The model under review builds one solid part; all positions refer to its coordinate system, in mm. Face numbers are marked on the shaded views. A direction names the side the tool comes from. Round coordinates to 2 decimals unless told otherwise and drop trailing zeros. Write each loop counter-clockwise with the first axis right and the second up, starting at its lowest first coordinate (ties: lowest second). Pieces come first, ordered by that corner, then holes. Notation, with made-up numbers: M 53.5,-9 L 105.5,-9 A16 ccw 105.5,12 Z; hole C 0,4.5 d5. An arc over 180 degrees is marked long. Write item = value, one per line. Start each with the question number.
Item 1: The part is to be moulded in two halves that separate along X. For the marked faces 4, 5 and 6, say which applies: +X half, -X half, draft (parallel to the pull), parting line (faces both ways), or undercut.
Item 2: Take a section at A-A, the plane x = 0. Give the boundary of the cut face in (y, z), plus the area to 3 significant figures.
Item 3: Take a section at B-B, the plane z = 0.45. Give the boundary of the cut face in (x, y) (3 decimals).
Item 4: Tool access review of the marked faces 1, 2 and 3: name each direction out of +Z, -Z, +X, -X, +Y, -Y from which nothing blocks a thin tool from reaching the whole face with its end or side.
Item 5: Take a section at C-C, the plane y = 0. Give the boundary of the cut face in (x, z), plus the area to 3 significant figures.
Item 6: Take a section at D-D, the plane x = 27.5. Give the boundary of the cut face in (y, z).
Item 7: For pin 1 Ø1.5 at (x, z) = (30, 0.5) entering from -Y, flat-tipped, find the tip position at first contact; note if it passes through.
Item 8: To check wall thickness, follow line 1 along X through (y, z) = (0.25, 1.5); line 2 along Z through (x, y) = (9, 2.75); line 3 along Y through (x, z) = (32, -0.15). State the ranges of each line that lie inside material, in increasing order.
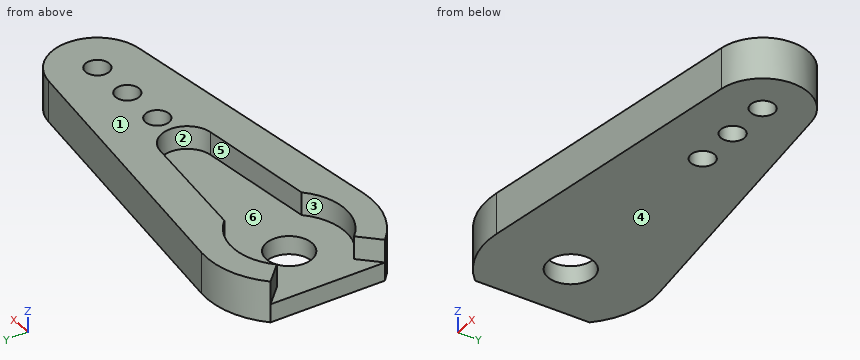
from build123d import *

# Parameters (mm, degrees)
MAIN_DEPTH            = 2.5
ORIGINALBRACKET_START = 2
ESQUISSE2_R           = 2.5
ORIGINALBRACKET_DEPTH = 2
ESQUISSE3_R           = 1.3
FIXINGHOLE_DEPTH      = 39.34383914


with BuildPart() as part:
    # Esquisse1 → Main (new body)
    with BuildSketch(Plane.XY):
        with BuildLine():
            Line((-4.375785644, 4.25), (-6.426543071, 6.300757427))
            ThreePointArc((-6.426543071, 6.300757427), (-2.958723408, 8.499762102), (1.125, 8.929410675))
            Line((1.125, 8.929410675), (32.625, 4.960783708))
            ThreePointArc((32.625, 4.960783708), (37, 0), (32.625, -4.960783708))
            Line((32.625, -4.960783708), (1.125, -8.929410675))
            ThreePointArc((1.125, -8.929410675), (-2.958723408, -8.499762102), (-6.426543071, -6.300757427))
            Line((-6.426543071, -6.300757427), (-4.375785644, -4.25))
            ThreePointArc((-4.375785644, -4.25), (0, -6.1), (4.375785644, -4.25))
            Line((4.375785644, -4.25), (17.31559729, -2.78215714))
            ThreePointArc((17.31559729, -2.78215714), (19.8, 0), (17.31559729, 2.78215714))
            Line((17.31559729, 2.78215714), (4.375785644, 4.25))
            ThreePointArc((4.375785644, 4.25), (0, 6.1), (-4.375785644, 4.25))
        make_face()
    extrude(amount=MAIN_DEPTH)

    # Esquisse2 → OriginalBracket (add)
    with BuildSketch(Plane(origin=(0, 0, 0), x_dir=(-1, 0, 0), z_dir=(0, 0, -1)).offset(ORIGINALBRACKET_START)):
        with BuildLine():
            Line((-1.125, -8.929410675), (-32.625, -4.960783708))
            ThreePointArc((-32.625, -4.960783708), (-37, 0), (-32.625, 4.960783708))
            Line((-32.625, 4.960783708), (-1.125, 8.929410675))
            ThreePointArc((-1.125, 8.929410675), (2.958723408, 8.499762102), (6.426543071, 6.300757427))
            Line((6.426543071, 6.300757427), (6.426543071, -6.300757427))
            ThreePointArc((6.426543071, -6.300757427), (2.958723408, -8.499762102), (-1.125, -8.929410675))
        make_face()
        Circle(ESQUISSE2_R, mode=Mode.SUBTRACT)
    extrude(amount=-ORIGINALBRACKET_DEPTH)

    # Esquisse3 → FixingHole (cut, through all)
    with BuildSketch(Plane.XY.offset(2.5)):
        with Locations((32, 0)):
            Circle(ESQUISSE3_R)
        with Locations((22, 0)):
            Circle(ESQUISSE3_R)
        with Locations((27, 0)):
            Circle(ESQUISSE3_R)
    extrude(amount=-FIXINGHOLE_DEPTH, mode=Mode.SUBTRACT)


solid = part.part
Response values:
q1.face_4 = draft
q1.face_5 = -X half
q1.face_6 = undercut
q2.outline = M -9,-2 L -2.5,-2 L -2.5,0 L -6.1,0 L -6.1,2.5 L -9,2.5 Z; M 2.5,-2 L 9,-2 L 9,2.5 L 6.1,2.5 L 6.1,0 L 2.5,0 Z
q2.area = 40.5 mm2
q3.outline = M -6.427,-6.301 A9 ccw 1.125,-8.929 L 32.625,-4.961 A5 ccw 32.625,4.961 L 1.125,8.929 A9 ccw -6.427,6.301 L -4.376,4.25 A6.1 cw 4.376,4.25 L 17.316,2.782 A2.8 cw 17.316,-2.782 L 4.376,-4.25 A6.1 cw -4.376,-4.25 Z; hole C 22,0 d2.6; hole C 27,0 d2.6; hole C 32,0 d2.6
q4.face_1 = +Z, +X, -X, +Y, -Y
q4.face_2 = +Z, -X
q4.face_3 = +Z
q5.outline = M -6.43,-2 L -2.5,-2 L -2.5,0 L -6.43,0 Z; M 2.5,-2 L 20.7,-2 L 20.7,2.5 L 19.8,2.5 L 19.8,0 L 2.5,0 Z; M 23.3,-2 L 25.7,-2 L 25.7,2.5 L 23.3,2.5 Z; M 28.3,-2 L 30.7,-2 L 30.7,2.5 L 28.3,2.5 Z; M 33.3,-2 L 37,-2 L 37,2.5 L 33.3,2.5 Z
q5.area = 84.8 mm2
q6.outline = M -5.61,-2 L -1.2,-2 L -1.2,2.5 L -5.61,2.5 Z; M 1.2,-2 L 5.61,-2 L 5.61,2.5 L 1.2,2.5 Z
q7.pin_1 = -5.39
q8.line_1 = 19.79 to 20.72, 23.28 to 25.72, 28.28 to 30.72, 33.28 to 36.99
q8.line_2 = -2 to 0
q8.line_3 = -5.04 to -1.3, 1.3 to 5.04
